Geometry: see drawing. Coordinates: mm, zero at the bounding-box minimum. Round coordinates to 2 decimals unless told otherwise and drop trailing zeros. Loops run counter-clockwise (first coordinate to the right, second up) from the corner with the lowest first, then second, coordinate; pieces in that order, holes last. Notation, with made-up numbers: M -38.75,19.25 L 6.25,19.25 A16 cw 6.25,33.25 Z; hole C -29,47.5 d11. An arc over 180 degrees is marked long. Answer as a JSON object with one key per item and string values.
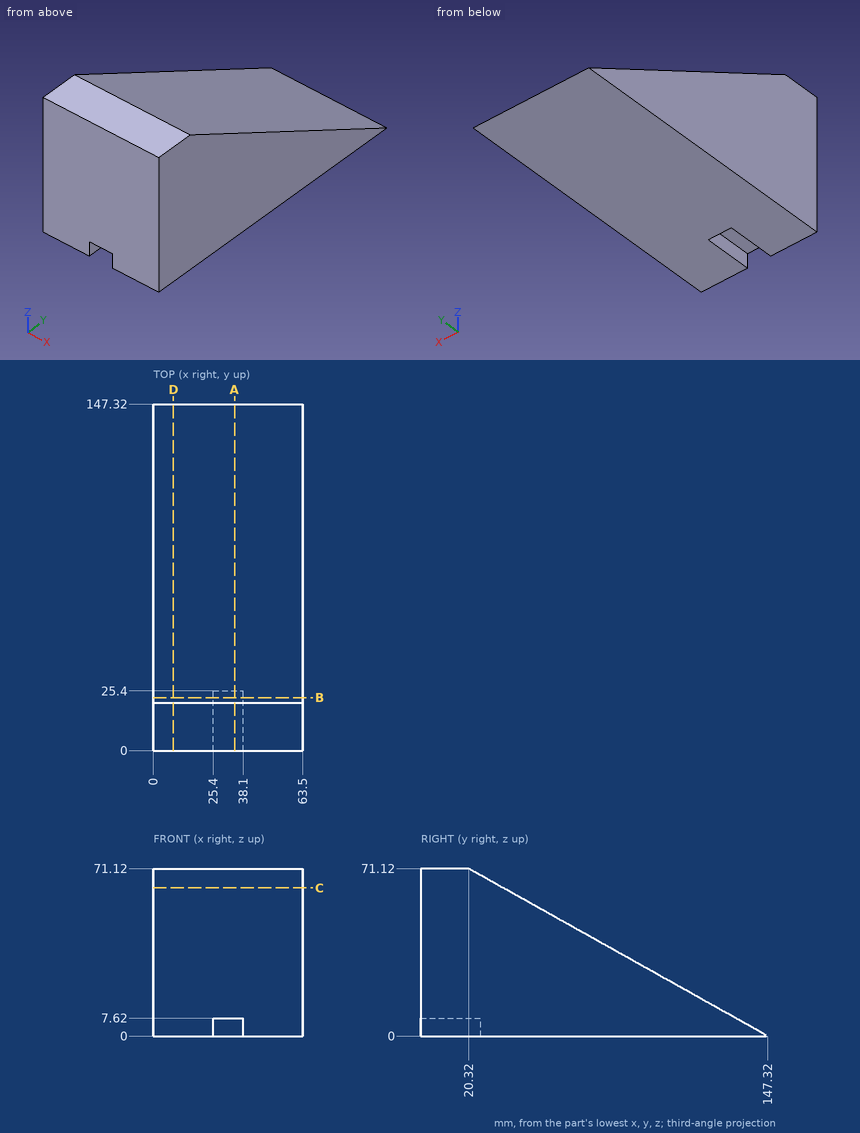
1) Section query D-D (x = 8.5). Return the cut outline in (y, z), and give its area (3 significant figures).
Results:
{"outline": "M 0,0 L 147.32,0 L 20.32,71.12 L 0,71.12 Z", "area": "5,960 mm2"}
2) Section query A-A (x = 34.5). Return the cut outline in (y, z), and give its area (3 significant figures).
Results:
{"outline": "M 0,7.62 L 25.4,7.62 L 25.4,0 L 147.32,0 L 20.32,71.12 L 0,71.12 Z", "area": "5,770 mm2"}
3) Ray query, line 1 (Z direction, x = 21.5, y = 102); line 2 (Z direction, x = 37, y = 140); line 3 (Y direction, x = 38, z = 63). Return the intervals inside material, ascending.
Results:
{"line 1": "0 to 25.38", "line 2": "0 to 4.1", "line 3": "0 to 34.82"}
4) Section query C-C (z = 63). Return the cut outline in (x, y).
Results:
{"outline": "M 0,0 L 63.5,0 L 63.5,34.82 L 0,34.82 Z"}
5) Pin query (flat end, axial travel): P1, Ø10, axis at x = 7.5, z = 32, coming from the +Y side; P2, Ø8, axis at x = 44, z = 25.5, coming from the -Y side. Return the tip coordinate at first contact, or that it passes through.
Results:
{"P1": "y = 99.11", "P2": "y = 0"}
6) Section query B-B (y = 22.5). Return the cut outline in (x, z), and give its area (3 significant figures).
Results:
{"outline": "M 0,0 L 25.4,0 L 25.4,7.62 L 38.1,7.62 L 38.1,0 L 63.5,0 L 63.5,69.9 L 0,69.9 Z", "area": "4,340 mm2"}
